Input: part model. Units: mm. Frame: model coordinates. Give positions to 0.01 mm unless a question says otherwise; leave off trailing zeros. Use a Markdown table: item, result.
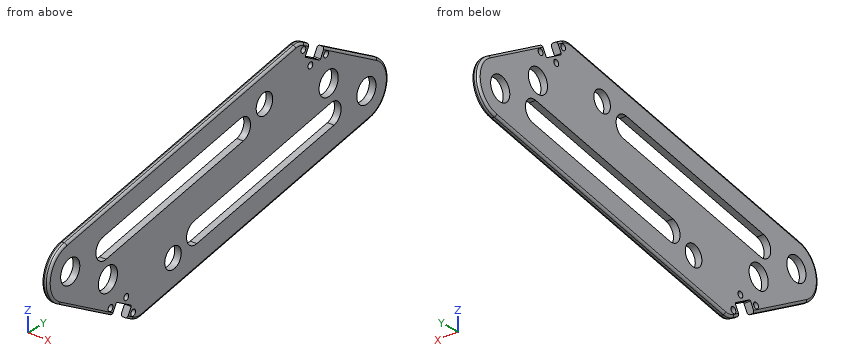
from build123d import *

# Parameters (mm, degrees)
SKETCH_2_R          = 9.5
SKETCH_2_R_2        = 11
EXTRUDE_1_DEPTH     = 6
CUT_EXTRUDE_1_DEPTH = 10
FILLET_1_R          = 25
SKETCH_4_R          = 2.75
CUT_EXTRUDE_2_DEPTH = 10
FILLET_2_R          = 15
FILLET_3_R          = 1
FILLET_4_R          = 2


with BuildPart() as part:
    # 草图2 → 凸台-拉伸1 (new body)
    with BuildSketch(Plane(origin=(0, 0, 0), x_dir=(0, 0, -1), z_dir=(1, 0, 0))):
        Polygon((12.494318662, 71.640794729), (-72.751567756, -76.009411684), (-12.535755442, -411.712565336), (72.916857811, -263.704297543), align=None)
        with Locations((-40, -117)):
            Circle(SKETCH_2_R, mode=Mode.SUBTRACT)
        with Locations((25, -296.698729811)):
            Circle(SKETCH_2_R_2, mode=Mode.SUBTRACT)
        with Locations((0, -340)):
            Circle(SKETCH_2_R_2, mode=Mode.SUBTRACT)
        with Locations((-25, -43.301270189)):
            Circle(SKETCH_2_R_2, mode=Mode.SUBTRACT)
        with Locations((40, -222)):
            Circle(SKETCH_2_R, mode=Mode.SUBTRACT)
        Circle(SKETCH_2_R_2, mode=Mode.SUBTRACT)
    extrude(amount=EXTRUDE_1_DEPTH)

    # 草图3 → 切除-拉伸1 (cut)
    with BuildSketch(Plane(origin=(6, 0, 0), x_dir=(0, 0, -1), z_dir=(1, 0, 0))):
        with BuildLine():
            Line((-20.40575236, -141.278289439), (7.842954525, -298.764830322))
            ThreePointArc((7.842954525, -298.764830322), (-0.2344101, -310.373283308), (-11.842863085, -302.295918683))
            Line((-11.842863085, -302.295918683), (-40.09156997, -144.8093778))
            ThreePointArc((-40.09156997, -144.8093778), (-32.014205345, -133.200924814), (-20.40575236, -141.278289439))
        make_face()
        with BuildLine():
            Line((11.783440235, -37.201240644), (40.155401092, -194.665623401))
            ThreePointArc((40.155401092, -194.665623401), (32.087124724, -206.280394877), (20.472353248, -198.212118508))
            Line((20.472353248, -198.212118508), (-7.89960761, -40.747735751))
            ThreePointArc((-7.89960761, -40.747735751), (0.168668759, -29.132964275), (11.783440235, -37.201240644))
        make_face()
    extrude(amount=-CUT_EXTRUDE_1_DEPTH, mode=Mode.SUBTRACT)

    # 圆角1
    fillet_1_edges = [part.edges().sort_by_distance(p)[0] for p in [
        (3, -411.712565336, 12.535755442),
        (3, 71.640794729, -12.494318662),
    ]]
    fillet(fillet_1_edges, radius=FILLET_1_R)

    # 草图4 → 切除-拉伸2 (cut)
    with BuildSketch(Plane(origin=(6, 0, 0), x_dir=(0, 0, -1), z_dir=(1, 0, 0))):
        with Locations((-49.820508076, -46.291651246)):
            Circle(SKETCH_4_R)
        with Locations((-64.820508076, -72.27241336)):
            Circle(SKETCH_4_R)
        with Locations((-48.660254038, -64.282032303)):
            Circle(SKETCH_4_R)
        with Locations((48.660254038, -275.717967697)):
            Circle(SKETCH_4_R)
        with Locations((49.820508076, -293.708348754)):
            Circle(SKETCH_4_R)
        with Locations((64.820508076, -267.72758664)):
            Circle(SKETCH_4_R)
        Polygon((-66.650635095, -65.442286341), (-56.650635095, -48.121778265), (-47.990381057, -53.121778265), (-57.990381057, -70.442286341), align=None)
        Polygon((47.990381057, -286.878221735), (57.990381057, -269.557713659), (66.650635095, -274.557713659), (56.650635095, -291.878221735), align=None)
    extrude(amount=-CUT_EXTRUDE_2_DEPTH, mode=Mode.SUBTRACT)

    # 圆角2
    fillet_2_edges = [part.edges().sort_by_distance(p)[0] for p in [
        (3, -263.704297543, -72.916857811),
        (3, -76.009411684, 72.751567756),
    ]]
    fillet(fillet_2_edges, radius=FILLET_2_R)

    # 圆角3
    fillet_3_edges = [part.edges().sort_by_distance(p)[0] for p in [
        (3, -286.878221735, -47.990381057),
        (3, -269.557713659, -57.990381057),
        (3, -53.121778265, 47.990381057),
        (3, -70.442286341, 57.990381057),
    ]]
    fillet(fillet_3_edges, radius=FILLET_3_R)

    # 圆角4
    fillet_4_edges = [part.edges().sort_by_distance(p)[0] for p in [
        (0, -212.910875987, 48.195251289),
        (6, -212.910875987, 48.195251289),
        (0, -126.933453974, -48.273462573),
        (0, -263.537032824, -71.957783708),
        (0, -76.176657925, 71.794811932),
        (6, -126.933453974, -48.273462573),
        (6, -263.537032824, -71.957783708),
        (6, -76.176657925, 71.794811932),
        (0, -322.189110868, -39.150635095),
        (6, -322.189110868, -39.150635095),
        (0, -17.810889132, 39.150635095),
        (0, 24.628257085, -4.295224436),
        (0, -364.626574291, 4.304862213),
        (6, -17.810889132, 39.150635095),
        (6, 24.628257085, -4.295224436),
        (6, -364.626574291, 4.304862213),
        (6, -271.508805911, -68.410922804),
        (0, -271.508805911, -68.410922804),
        (6, -68.350930797, 68.329941754),
        (0, -68.350930797, 68.329941754),
    ]]
    fillet(fillet_4_edges, radius=FILLET_4_R)


solid = part.part
1. Section query A-A (y = -117). State how many separate pieces and enclosed holes the cut face has, then the cut area to 3 significant figures.
Response:
| item | result |
|---|---|
| separate pieces | 3 |
| enclosed holes | 0 |
| area | 432 mm^2 |
2. Material intervals for line 1 along Z through (x, y) = (5.75, -300.5) (3 decimals); line 2 along Z through (x, y) = (1, -149.5); line 3 along Z through (x, y) = (2.75, -348.5), sorted ascending.
Response:
| item | result |
|---|---|
| line 1 | z = -50.481 to -35.322, -14.678 to -8, 12.165 to 31.436 |
| line 2 | z = -52.07 to -32.02, -11.7 to 18.93, 39.25 to 59.3 |
| line 3 | z = -23.96 to -6.98, 6.98 to 23.51 |
3. Pin query (flat end, axial travel): pin 1 (20 mm diameter, centred on y = 0, z = 0, fed in from +X) (3 decimals); pin 2 (1.5 mm diameter, centred on x = 3, z = 50.5, fed in from +Y). Return the tip coordinate at first contact, or that it passes through.
Response:
| item | result |
|---|---|
| pin 1 | passes through |
| pin 2 | stops at y = -36.17 |
